```python
from build123d import *

# Parameters (mm, degrees)
SKETCH1_W                      = 350
SKETCH1_H                      = 340
BASE_FLANGE1_DEPTH             = 1.51892
M3_CLEARANCE_HOLE1_D           = 3.6
M4_CLEARANCE_HOLE1_D           = 4.8
SKETCH41_W                     = 340
SKETCH41_H                     = 1.51892
BOSS_EXTRUDE4_DEPTH            = 1.905
SKETCH42_W                     = 340
SKETCH42_H                     = 1.51892
BOSS_EXTRUDE5_DEPTH            = 1.905
CUT_EXTRUDE3_DEPTH             = 1.51892
SKETCH51_R                     = 1.55
SKETCH51_R_2                   = 1.27
SKETCH51_W                     = 46.695999999
SKETCH51_H                     = 7.064
SKETCH51_W_2                   = 18.24
CUT_EXTRUDE4_DEPTH             = 1.51892
CHAMFER1_SIZE                  = 11
SKETCH62_W                     = 25
SKETCH62_H                     = 10
SKETCH62_W_2                   = 7
CUT_EXTRUDE6_DEPTH             = 1.51892
FILLET4_R                      = 3.5
EDGE_FLANGE4_STRIP_W           = 6.83768
EDGE_FLANGE4_STRIP_H           = 1.51892
EDGE_FLANGE4_STRIP_CUT_DEPTH   = 331.81
EDGE_FLANGE4_STRIP_2_W         = 6.83768
EDGE_FLANGE4_STRIP_2_H         = 1.51892
EDGE_FLANGE4_STRIP_CUT_2_DEPTH = 322.430780628
EDGE_FLANGE4_DEPTH             = 331.81
EDGE_FLANGE4_BEND_DEPTH        = 322.430780628
M2_CLEARANCE_HOLE1_D           = 2.4
M4_CLEARANCE_HOLE3_D           = 4.5
M4_CLEARANCE_HOLE3_DEPTH       = 11.5189
M4_CLEARANCE_HOLE3_TIP         = 1.351936393
M4_CLEARANCE_HOLE4_D           = 4.5
M4_CLEARANCE_HOLE4_DEPTH       = 11.5189
M4_CLEARANCE_HOLE4_TIP         = 1.351936393


# Sheet-metal steps are written as plain solids
with BuildPart() as part:
    # Sketch1 → Base-Flange1 (new body)
    with BuildSketch(Plane(origin=(0, 0, 0), x_dir=(1, 0, 0), z_dir=(0, 1, 0))):
        with Locations((0, 5)):
            Rectangle(SKETCH1_W, SKETCH1_H)
    extrude(amount=-BASE_FLANGE1_DEPTH)

    # M3 Clearance Hole1 (through all)
    with Locations(Plane(origin=(0, 0, 0), x_dir=(1, 0, 0), z_dir=(0, 1, 0))):
        with Locations((-105, 105), (105, 105), (105, -105), (-105, -105)):
            Hole(M3_CLEARANCE_HOLE1_D / 2)

    # M4 Clearance Hole1 (through all)
    with Locations(Plane(origin=(0, -1.51892, 0), x_dir=(-1, 0, 0), z_dir=(0, -1, 0))):
        with Locations((-161.000000003, -155.500000003), (31.25, 165), (8.75, 165), (138.500000003, -155.500000003), (161.000000003, -155.500000003), (-138.500000003, -155.500000003)):
            Hole(M4_CLEARANCE_HOLE1_D / 2)

    # Sketch41 → Boss-Extrude4 (add)
    with BuildSketch(Plane(origin=(175, 0, 0), x_dir=(0, 0, -1), z_dir=(1, 0, 0))):
        with Locations((5, -0.75946)):
            Rectangle(SKETCH41_W, SKETCH41_H)
    extrude(amount=BOSS_EXTRUDE4_DEPTH)

    # Sketch42 → Boss-Extrude5 (add)
    with BuildSketch(Plane.ZY.offset(175)):
        with Locations((-5, -0.75946)):
            Rectangle(SKETCH42_W, SKETCH42_H)
    extrude(amount=BOSS_EXTRUDE5_DEPTH)

    # Sketch50 → Cut-Extrude3 (cut)
    with BuildSketch(Plane(origin=(0, 0, 0), x_dir=(1, 0, 0), z_dir=(0, 1, 0))):
        Polygon((-176.905, 175), (-168.143593544, 175), (-176.905, 159.824798873), align=None)
        Polygon((168.143593544, 175), (176.905, 159.824798873), (176.905, 175), align=None)
    extrude(amount=-CUT_EXTRUDE3_DEPTH, mode=Mode.SUBTRACT)

    # Sketch51 → Cut-Extrude4 (cut)
    with BuildSketch(Plane(origin=(0, 0, 0), x_dir=(1, 0, 0), z_dir=(0, 1, 0))):
        with Locations(Location((0, 104.499999999, 0), (0, 0, 270))):
            Circle(SKETCH51_R)
        with Locations(Location((0, 0, 0), (0, 0, 270))):
            Circle(SKETCH51_R_2)
        with Locations((26.760000001, 100.904)):
            Rectangle(SKETCH51_W, SKETCH51_H)
        with Locations((-16.67, 100.904)):
            Rectangle(SKETCH51_W_2, SKETCH51_H)
    extrude(amount=-CUT_EXTRUDE4_DEPTH, mode=Mode.SUBTRACT)

    # Chamfer1
    chamfer1_edges = [part.edges().sort_by_distance(p)[0] for p in [
        (176.905, -0.75946, 165),
        (-176.905, -0.75946, 165),
    ]]
    chamfer(chamfer1_edges, length=CHAMFER1_SIZE)

    # Sketch62 → Cut-Extrude6 (cut)
    with BuildSketch(Plane(origin=(0, 0, 0), x_dir=(1, 0, 0), z_dir=(0, 1, 0))):
        with Locations((-1.587999999, 95.904)):
            Rectangle(SKETCH62_W, SKETCH62_H)
        with Locations((0, 5)):
            Rectangle(SKETCH62_W_2, SKETCH62_H)
    extrude(amount=-CUT_EXTRUDE6_DEPTH, mode=Mode.SUBTRACT)

    # Fillet4
    fillet4_edges = [part.edges().sort_by_distance(p)[0] for p in [
        (-14.087999999, -0.75946, -97.372),
        (-7.55, -0.75946, -100.904),
        (10.912000001, -0.75946, -97.372),
        (3.412000001, -0.75946, -100.904),
    ]]
    fillet(fillet4_edges, radius=FILLET4_R)

    # Edge-Flange4 strip (across the edge) → Edge-Flange4 strip cut (cut)
    with BuildSketch(Plane(origin=(165.905, -1.51892, 165), x_dir=(0, 0, -1), z_dir=(-1, 0, 0))):
        with Locations((-1.51892, -0.75946)):
            Rectangle(EDGE_FLANGE4_STRIP_W, EDGE_FLANGE4_STRIP_H)
    extrude(amount=EDGE_FLANGE4_STRIP_CUT_DEPTH, mode=Mode.SUBTRACT)

    # Edge-Flange4 strip 2 (across the edge) → Edge-Flange4 strip cut 2 (cut)
    with BuildSketch(Plane(origin=(-161.215390314, -1.51892, -175), x_dir=(0, 0, 1), z_dir=(1, 0, 0))):
        with Locations((-1.51892, -0.75946)):
            Rectangle(EDGE_FLANGE4_STRIP_2_W, EDGE_FLANGE4_STRIP_2_H)
    extrude(amount=EDGE_FLANGE4_STRIP_CUT_2_DEPTH, mode=Mode.SUBTRACT)

    # Edge-Flange4 section (across the edge) → Edge-Flange4 (add)
    with BuildSketch(Plane(origin=(165.905, -1.51892, 165), x_dir=(0, 0, -1), z_dir=(-1, 0, 0))):
        with BuildLine():
            Line((0, 0.381), (0, 10))
            Line((0, 10), (1.51892, 10))
            Line((1.51892, 10), (1.51892, 0.381))
            ThreePointArc((1.51892, 0.381), (1.630512316, 0.111592316), (1.89992, 0))
            Line((1.89992, 0), (1.89992, -1.51892))
            ThreePointArc((1.89992, -1.51892), (0.556473684, -0.962446316), (0, 0.381))
        make_face()
    extrude(amount=EDGE_FLANGE4_DEPTH)

    # Edge-Flange4 section 2 (across the edge) → Edge-Flange4 bend (add)
    with BuildSketch(Plane(origin=(-161.215390314, -1.51892, -175), x_dir=(0, 0, 1), z_dir=(1, 0, 0))):
        with BuildLine():
            Line((0, 0.381), (0, 10))
            Line((0, 10), (1.51892, 10))
            Line((1.51892, 10), (1.51892, 0.381))
            ThreePointArc((1.51892, 0.381), (1.630512316, 0.111592316), (1.89992, 0))
            Line((1.89992, 0), (1.89992, -1.51892))
            ThreePointArc((1.89992, -1.51892), (0.556473684, -0.962446316), (0, 0.381))
        make_face()
    extrude(amount=EDGE_FLANGE4_BEND_DEPTH)

    # M2 Clearance Hole1 (through all)
    with Locations(Plane(origin=(0, 0, 0), x_dir=(1, 0, 0), z_dir=(0, 1, 0))):
        with Locations((-94.05, 167), (-75, 167), (75, 167), (94.05, 167)):
            Hole(M2_CLEARANCE_HOLE1_D / 2)

    # M4 Clearance Hole3
    with Locations(Plane.XY.offset(165)):
        with Locations((132.349919958, -7), (-132.349919958, -7)):
            Hole(M4_CLEARANCE_HOLE3_D / 2, depth=M4_CLEARANCE_HOLE3_DEPTH)
            with Locations((0, 0, -(M4_CLEARANCE_HOLE3_DEPTH + M4_CLEARANCE_HOLE3_TIP / 2))):  # 118° drill point
                Cone(0, M4_CLEARANCE_HOLE3_D / 2, M4_CLEARANCE_HOLE3_TIP, mode=Mode.SUBTRACT)

    # M4 Clearance Hole4
    with Locations(Plane(origin=(0, 0, -175), x_dir=(-1, 0, 0), z_dir=(0, 0, -1))):
        with Locations((0, -6.5)):
            Hole(M4_CLEARANCE_HOLE4_D / 2, depth=M4_CLEARANCE_HOLE4_DEPTH)
            with Locations((0, 0, -(M4_CLEARANCE_HOLE4_DEPTH + M4_CLEARANCE_HOLE4_TIP / 2))):  # 118° drill point
                Cone(0, M4_CLEARANCE_HOLE4_D / 2, M4_CLEARANCE_HOLE4_TIP, mode=Mode.SUBTRACT)


solid = part.part
```
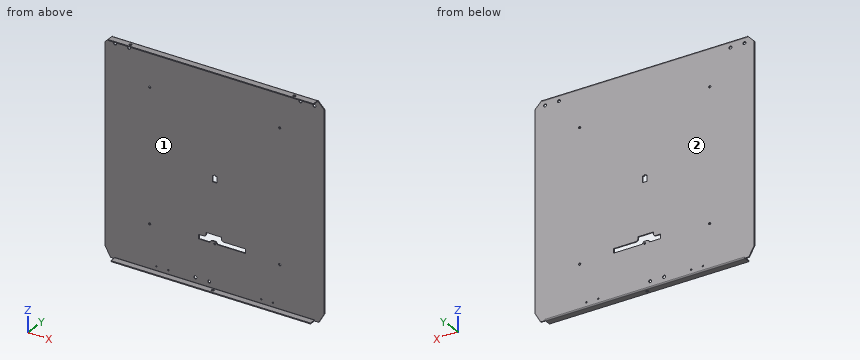
Can you work these out from the model? Positions are in its coordinate system, mm. Face numbers are marked on the shaded views. Give positions to 0.01 mm unless a question says otherwise; leave off trailing zeros. Order: outer loops, then holes, each group sorted by start corner. A loop starts at its lowest first (then second) coordinate and runs counter-clockwise, first axis right, second up. Notation, with made-up numbers: (55.25, 29.25) - (96.25, 29.25) arc R22 cw to (96.25, 44.25) - close; hole circle Ø11 at (-38, -14.75). An arc over 180 degrees is marked (long way). Use a Markdown table: item, result. Add a question column.
Q1. If we section it at B-B on x = -40: Write out the boundary of the cut face in (y, z), plus the area to 3 significant figures.
Q2. If we section it at C-C on z = -115: Write out the boundary of the cut face in (x, y) (3 decimals).
Q3. Please list where these lines run through material, in increasing order: line 1 along X through (y, z) = (-0.35, -104.5) (3 decimals); line 2 along Z through (x, y) = (116.5, -6.5); line 3 along Y through (x, z) = (-44, -105).
Q4. If we mould it in two halves opening along Z, with no side actions, what happens to the marked faces 1 and 2? For each: released by +Z, released by -Z, zero draft, split by the parting line, or undercut.
Q5. I'm going to push flat-ended pins straight in: pin 1 (0.8 mm diameter, centred on x = 28.5, y = -0.5, fed in from -Z); pin 2 (1.2 mm diameter, centred on x = 24.5, y = -0.5, fed in from +Z); pin 3 (0.5 mm diameter, centred on x = -23, y = -1, fed in from -Z). Where does each tip first touch, or does it pass through?
Q6. If we section it at A-A on x = 22.5: Write out the boundary of the cut face in (y, z).
Answers follow:
| question | item | result |
|---|---|---|
| 1 | outline | (-11.52, -175) - (-1.9, -175) arc R1.9 ccw to (0, -173.1) - (0, 163.1) arc R1.9 ccw to (-1.9, 165) - (-11.52, 165) - (-11.52, 163.48) - (-1.9, 163.48) arc R0.38 cw to (-1.52, 163.1) - (-1.52, -173.1) arc R0.38 cw to (-1.9, -173.48) - (-11.52, -173.48) - close |
| 1 | area | 545 mm^2 |
| 2 | outline | (-176.905, -1.519) - (176.905, -1.519) - (176.905, 0) - (-176.905, 0) - close |
| 3 | line 1 | x = -176.905 to -106.729, -103.271 to -1.55, 1.55 to 103.271, 106.729 to 176.905 |
| 3 | line 2 | z = -175 to -173.48, 163.48 to 165 |
| 3 | line 3 | y = -1.52 to 0 |
| 4 | face 1 | undercut |
| 4 | face 2 | zero draft |
| 5 | pin 1 | stops at z = -174.72 |
| 5 | pin 2 | stops at z = 164.82 |
| 5 | pin 3 | stops at z = -174.89 |
| 6 | outline | (-11.52, -175) - (-1.9, -175) arc R1.9 ccw to (0, -173.1) - (0, -104.44) - (-1.52, -104.44) - (-1.52, -173.1) arc R0.38 cw to (-1.9, -173.48) - (-11.52, -173.48) - close; (-11.52, 163.48) - (-1.9, 163.48) arc R0.38 cw to (-1.52, 163.1) - (-1.52, -97.37) - (0, -97.37) - (0, 163.1) arc R1.9 ccw to (-1.9, 165) - (-11.52, 165) - close |
